CAD build for the part. Positions are in the model's coordinates, mm. Coordinates: 2 decimals unless noted, no trailing zeros. Write each loop counter-clockwise with the first axis right and the second up, starting at its lowest first coordinate (ties: lowest second). Pieces come first, ordered by that corner, then holes. Notation, with made-up numbers: M 68,51.5 L 76,51.5 A16 ccw 76,67.5 Z; hole C 78,-35.5 d1. An arc over 180 degrees is marked long. Answer as CSV lines item,"result". Start each with the question number.
```python
from build123d import *

# Parameters (mm, degrees)
SKETCH_1_W          = 50
SKETCH_1_H          = 22.75
SKETCH_1_H_2        = 35
SKETCH_1_W_2        = 40
SKETCH_1_H_3        = 120
SKETCH_1_W_3        = 25
SKETCH_1_H_4        = 90
SKETCH_1_W_4        = 6
SKETCH_1_H_5        = 18
EXTRUDE_1_DEPTH     = 5
SKETCH_2_R          = 1.5
CUT_EXTRUDE_1_DEPTH = 10
SKETCH_3_R          = 1.5
CUT_EXTRUDE_2_DEPTH = 10
SKETCH_4_R          = 1.5
CUT_EXTRUDE_3_DEPTH = 10
SKETCH_5_R          = 1.5
CUT_EXTRUDE_4_DEPTH = 24
SKETCH_6_R          = 1.6
CUT_EXTRUDE_5_DEPTH = 10
SKETCH_7_W          = 3
SKETCH_7_H          = 172
CUT_EXTRUDE_6_DEPTH = 10
SKETCH_9_R          = 1.5
CUT_EXTRUDE_7_DEPTH = 5
SKETCH_10_R         = 1.35
CUT_EXTRUDE_8_DEPTH = 10


with BuildPart() as part:
    # 草图1 → 凸台-拉伸1 (new body)
    with BuildSketch(Plane.XY):
        Polygon((-105.75, 86), (-105.75, 70), (-105.75, -86), (105.75, -86), (105.75, 86), align=None)
        with Locations((-50.75, 58.625)):
            Rectangle(SKETCH_1_W, SKETCH_1_H, mode=Mode.SUBTRACT)
        with Locations((-50.75, 22.5)):
            Rectangle(SKETCH_1_W, SKETCH_1_H_2, mode=Mode.SUBTRACT)
        with Locations((-50.75, -58.625)):
            Rectangle(SKETCH_1_W, SKETCH_1_H, mode=Mode.SUBTRACT)
        with Locations((26.25, 0)):
            Rectangle(SKETCH_1_W_2, SKETCH_1_H_3, mode=Mode.SUBTRACT)
        with Locations((74.75, 0)):
            Rectangle(SKETCH_1_W_3, SKETCH_1_H_4, mode=Mode.SUBTRACT)
        with Locations((-50.75, -22.5)):
            Rectangle(SKETCH_1_W, SKETCH_1_H_2, mode=Mode.SUBTRACT)
        with Locations((-12.75, -36)):
            Rectangle(SKETCH_1_W_4, SKETCH_1_H_5, mode=Mode.SUBTRACT)
        with Locations((-12.75, 36)):
            Rectangle(SKETCH_1_W_4, SKETCH_1_H_5, mode=Mode.SUBTRACT)
    extrude(amount=EXTRUDE_1_DEPTH)

    # 草图2 → 切除-拉伸1 (cut)
    with BuildSketch(Plane.XY.offset(5)):
        with Locations((97.05, 83)):
            Circle(SKETCH_2_R)
        with Locations((-93.55, 83)):
            Circle(SKETCH_2_R)
        with Locations((57.55, 83)):
            Circle(SKETCH_2_R)
        with Locations((-54.05, 83)):
            Circle(SKETCH_2_R)
        with Locations((57.55, -83)):
            Circle(SKETCH_2_R)
        with Locations((97.05, -83)):
            Circle(SKETCH_2_R)
        with Locations((-54.05, -83)):
            Circle(SKETCH_2_R)
        with Locations((-93.55, -83)):
            Circle(SKETCH_2_R)
    extrude(amount=-CUT_EXTRUDE_1_DEPTH, mode=Mode.SUBTRACT)

    # 草图3 → 切除-拉伸2 (cut)
    with BuildSketch(Plane.XY.offset(5)):
        with Locations((46.25, 75)):
            Circle(SKETCH_3_R)
        with Locations((46.25, -75)):
            Circle(SKETCH_3_R)
        with Locations((30.25, -75)):
            Circle(SKETCH_3_R)
        with Locations((30.25, 75)):
            Circle(SKETCH_3_R)
        with Locations((16.25, 75)):
            Circle(SKETCH_3_R)
        with Locations((16.25, -75)):
            Circle(SKETCH_3_R)
    extrude(amount=-CUT_EXTRUDE_2_DEPTH, mode=Mode.SUBTRACT)

    # 草图4 → 切除-拉伸3 (cut)
    with BuildSketch(Plane.XY.offset(5)):
        with Locations((-3.85, 75)):
            Circle(SKETCH_4_R)
        with Locations((-3.85, -75)):
            Circle(SKETCH_4_R)
    extrude(amount=-CUT_EXTRUDE_3_DEPTH, mode=Mode.SUBTRACT)

    # 草图5 → 切除-拉伸4 (cut)
    with BuildSketch(Plane.XY.offset(5)):
        with Locations((-17.75, 75)):
            Circle(SKETCH_5_R)
        with Locations((-83.25, 75)):
            Circle(SKETCH_5_R)
        with Locations((-83.25, -75)):
            Circle(SKETCH_5_R)
        with Locations((-17.75, -75)):
            Circle(SKETCH_5_R)
    extrude(amount=-CUT_EXTRUDE_4_DEPTH, mode=Mode.SUBTRACT)

    # 草图6 → 切除-拉伸5 (cut)
    with BuildSketch(Plane.XY.offset(5)):
        with Locations((-95.75, 45)):
            Circle(SKETCH_6_R)
        with Locations((-95.75, 0)):
            Circle(SKETCH_6_R)
        with Locations((-95.75, -45)):
            Circle(SKETCH_6_R)
    extrude(amount=-CUT_EXTRUDE_5_DEPTH, mode=Mode.SUBTRACT)

    # 草图7 → 切除-拉伸6 (cut)
    with BuildSketch(Plane.XY.offset(5)):
        with Locations((104.25, 0)):
            Rectangle(SKETCH_7_W, SKETCH_7_H)
    extrude(amount=-CUT_EXTRUDE_6_DEPTH, mode=Mode.SUBTRACT)

    # 草图9 → 切除-拉伸7 (cut)
    with BuildSketch(Plane.XY.offset(5)):
        with Locations((97.75, 10)):
            Circle(SKETCH_9_R)
    cut_extrude_7 = extrude(amount=-CUT_EXTRUDE_7_DEPTH, mode=Mode.SUBTRACT)

    # 镜向1: 切除-拉伸7 across plane
    add(cut_extrude_7.mirror(Plane.ZX), mode=Mode.SUBTRACT)

    # 草图10 → 切除-拉伸8 (cut)
    with BuildSketch(Plane.XY.offset(5)):
        with Locations((-95.75, 22.5)):
            Circle(SKETCH_10_R)
        with Locations((-95.75, -22.5)):
            Circle(SKETCH_10_R)
    extrude(amount=-CUT_EXTRUDE_8_DEPTH, mode=Mode.SUBTRACT)


solid = part.part
```
1) Two-plate mould, pull along Y, no slides. Class faces 1 (the flat face through (87.25, -1, 2)), 2 (the flat face through (-105.75, 1, 2)): pulls with the +Y half, pulls with the -Y half, needs draft (parallel to the pull), parting line crosses it, or undercut.
2) Probe L1, parallel to Y at x = -65, z = 0.85; L2, parallel to X at y = -10, z = 1.3; L3, parallel to Y at x = 16.25, z = 1.05. List the from-to ranges inside material, lowest first. Write a range as [from, to].
3) Band-saw the part on A-A, the plane y = -53. List the corners of the cut face in (x, z).
4) Band-saw the part on C-C, the plane z = 4. State how many separate pieces and enclosed holes the cut face has, plus the area to 3 significant figures.
5) Band-saw the part on B-B, the plane x = -65.5. List the corners of the cut face in (y, z).
Result sheet:
1,face 1,"undercut"
1,face 2,"needs draft"
2,L1,"y = [-86, -70], [-47.25, -40], [-5, 5], [40, 47.25], [70, 86]"
2,L2,"x = [-105.75, -75.75], [-25.75, 6.25], [46.25, 62.25], [87.25, 96.25], [99.25, 102.75]"
2,L3,"y = [-86, -76.5], [-73.5, -60], [60, 73.5], [76.5, 86]"
3,outline,"M -105.75,0 L -75.75,0 L -75.75,5 L -105.75,5 Z; M -25.75,0 L 6.25,0 L 6.25,5 L -25.75,5 Z; M 46.25,0 L 102.75,0 L 102.75,5 L 46.25,5 Z"
4,separate pieces,"1"
4,enclosed holes,"35"
4,area,"22,600 mm²"
5,outline,"M -86,0 L -70,0 L -70,5 L -86,5 Z; M -47.25,0 L -40,0 L -40,5 L -47.25,5 Z; M -5,0 L 5,0 L 5,5 L -5,5 Z; M 40,0 L 47.25,0 L 47.25,5 L 40,5 Z; M 70,0 L 86,0 L 86,5 L 70,5 Z"
